Geometry check sheet. Reference: the model listing, model coordinates, mm. A direction names the side the tool comes from. Round coordinates to 2 decimals unless told otherwise and drop trailing zeros. Order: outer loops, then holes, each group sorted by start corner. A loop starts at its lowest first (then second) coordinate and runs counter-clockwise, first axis right, second up.
```python
from build123d import *

# Parameters (mm, degrees)
F0_W      = 1663.7
F0_H      = 304.8
F1_DEPTH  = 19.05
F2_W      = 50.8
F2_H      = 19.05
F3_DEPTH  = 304.8
F4_W      = 1308.1
F4_H      = 19.05
F5_DEPTH  = 304.8
F7_DEPTH  = 19.05
F8_DEPTH  = 19.05
F9_DEPTH  = 19.05
F11_DEPTH = 19.05
F12_W     = 276.225
F12_H     = 19.05
F13_DEPTH = 304.8
F14_DEPTH = 50.8
F15_DEPTH = 304.8
F16_DEPTH = 304.8
F17_W     = 304.8
F17_H     = 19.05
F18_DEPTH = 152.4


with BuildPart() as f1:
    # F0 (on Front) → F1 (new body)
    with BuildSketch(Plane.XZ):
        Rectangle(F0_W, F0_H)
    extrude(amount=F1_DEPTH)

    # F2 (on face) → F3 (join)
    with BuildSketch(Plane.XZ.offset(19.05)):
        with Locations((806.45, -142.113)):
            Rectangle(F2_W, F2_H)
    extrude(amount=F3_DEPTH)

    # F4 (on face) → F5 (join)
    with BuildSketch(Plane.XZ.offset(19.05)):
        with Locations((-177.8, -142.113)):
            Rectangle(F4_W, F4_H)
    extrude(amount=F5_DEPTH)

    # F6 (on face) → F7 (join)
    with BuildSketch(Plane.XZ.offset(323.85)):
        Polygon((-831.85, 152.4), (-831.85, -151.638), (-831.85, -152.4), (831.85, -152.4), (831.85, 152.4), align=None)
    extrude(amount=F7_DEPTH)

    # F8 (cut): a face of the model
    f8_faces = [f1.faces().sort_by_distance(p)[0] for p in [
        (0, -333.375, 152.4),
    ]]
    extrude(f8_faces, amount=-F8_DEPTH, mode=Mode.SUBTRACT)

    # F9 (cut): a face of the model
    f9_faces = [f1.faces().sort_by_distance(p)[0] for p in [
        (0, -9.525, 152.4),
    ]]
    extrude(f9_faces, amount=-F9_DEPTH, mode=Mode.SUBTRACT)

    # F10 (on face) → F11 (join)
    with BuildSketch(Plane.XY.offset(133.35)):
        Polygon((831.85, -393.7), (831.85, -342.9), (831.85, -323.85), (831.85, -19.05), (781.05, -19.05), (781.05, -323.85), (425.45, -323.85), (425.45, -19.05), (361.95, -19.05), (361.95, -323.85), (-615.95, -323.85), (-679.45, -323.85), (-831.85, -323.85), (-831.85, -393.7), align=None)
        Polygon((781.05, -19.05), (831.85, -19.05), (831.85, 50.8), (-831.85, 50.8), (-831.85, -19.05), (-679.45, -19.05), (-679.45, -323.85), (-615.95, -323.85), (-615.95, -19.05), (361.95, -19.05), (425.45, -19.05), align=None)
    extrude(amount=F11_DEPTH)

    # F12 (on face) → F13 (join)
    with BuildSketch(Plane(origin=(0, -323.85, 0), x_dir=(-1, 0, 0), z_dir=(0, 1, 0))):
        with Locations((-617.5375, -142.113)):
            Rectangle(F12_W, F12_H)
    extrude(amount=F13_DEPTH)

    # F14 (cut): a face of the model
    f14_faces = [f1.faces().sort_by_distance(p)[0] for p in [
        (-831.85, -329.2396501742, 9.906),
    ]]
    extrude(f14_faces, amount=-F14_DEPTH, mode=Mode.SUBTRACT)

    # F15 (add): a face of the model
    f15_faces = [f1.faces().sort_by_distance(p)[0] for p in [
        (831.85, -329.2396501742, -152.019),
    ]]
    extrude(f15_faces, amount=F15_DEPTH)

    # F16 (cut): a face of the model
    f16_faces = [f1.faces().sort_by_distance(p)[0] for p in [
        (781.05, -171.45, 142.875),
    ]]
    extrude(f16_faces, amount=-F16_DEPTH, mode=Mode.SUBTRACT)

    # F17 (on face) → F18 (cut)
    with BuildSketch(Plane(origin=(-781.05, 0, 0), x_dir=(0, -1, 0), z_dir=(-1, 0, 0))):
        with Locations((171.45, -142.113)):
            Rectangle(F17_W, F17_H)
    extrude(amount=-F18_DEPTH, mode=Mode.SUBTRACT)


solid = f1.part
```
(1) Draft check along Y on faces 1 (the flat face through (956, -169, -132.588)), 2 (the flat face through (164, 0, -12)). Enter one of: released by +Y, released by -Y, zero draft, split by the parting line, or undercut.
Returned:
face 1: undercut
face 2: released by +Y
(2) Set-up check for faces 3 (the flat face through (-648, -169, 133.35)), 4 (the flat face through (-781.05, -2, 22)), 5 (the flat face through (164, -342.9, -12)), 6 (the flat face through (164, 25, 133.35)), 7 (the flat face through (619, -174, -132.588)): record each of +Z, -Z, +X, -X, +Y, -Y from which the full face is reachable in a straight line by a thin tool's end or side.
Returned:
face 3: +X, -X
face 4: +Z, -Z, -X, +Y, -Y
face 5: -Z, +X, -X, -Y
face 6: -Z, +X, -X, +Y
face 7: +Z, +X, -X
(3) Material ranges on line 1 (Y direction, x = -546, z = -29.5); line 2 (Z direction, x = 899, y = -307); line 3 (Z direction, x = -666, y = 23.5), recorded low to high.
Returned:
line 1: y = -342.9 to -323.85, -19.05 to 0
line 2: z = -151.64 to -132.59
line 3: z = 133.35 to 152.4
(4) Depth check by flat-ended pin: P1, Ø19, axis at x = 388.5, y = -160.5, coming from the -Z side; P2, Ø15, axis at y = -166.5, z = -144.5, coming from the -X side; P3, Ø8, axis at x = 130.5, z = -3, coming from the -Y side. Enter the tip coordinate at first touch or a pass-through.
Returned:
P1: stops at z = -151.64
P2: stops at x = -628.65
P3: stops at y = -342.9
(5) Sectioned sample at C-C, the plane x = 384. Record the cut outline in (y, z).
Returned:
outline: (-393.7, 133.35) - (-342.9, 133.35) - (-342.9, -152.4) - (-323.85, -152.4) - (-323.85, -151.64) - (-19.05, -151.64) - (-19.05, -152.4) - (0, -152.4) - (0, 133.35) - (50.8, 133.35) - (50.8, 152.4) - (-393.7, 152.4) - close; hole (-323.85, -132.59) - (-19.05, -132.59) - (-19.05, 133.35) - (-323.85, 133.35) - close
(6) Sectioned sample at A-A, the plane y = -134. Record the cut outline in (x, z) (3 decimals), and give its area (3 significant figures).
Returned:
outline: (-679.45, 133.35) - (-615.95, 133.35) - (-615.95, 152.4) - (-679.45, 152.4) - close; (-628.65, -151.638) - (476.25, -151.638) - (476.25, -132.588) - (-628.65, -132.588) - close; (361.95, 133.35) - (425.45, 133.35) - (425.45, 152.4) - (361.95, 152.4) - close; (479.425, -151.638) - (755.65, -151.638) - (755.65, -132.588) - (479.425, -132.588) - close; (781.05, -151.638) - (1136.65, -151.638) - (1136.65, -132.588) - (781.05, -132.588) - close; (1085.85, 133.35) - (1136.65, 133.35) - (1136.65, 152.4) - (1085.85, 152.4) - close
area: 36,500 mm2
(7) Sectioned sample at B-B, the plane z = -20.5. Record the cut outline in (x, y), and give its area (3 significant figures).
Returned:
outline: (-781.05, -342.9) - (1136.65, -342.9) - (1136.65, -323.85) - (-781.05, -323.85) - close; (-781.05, -19.05) - (1136.65, -19.05) - (1136.65, 0) - (-781.05, 0) - close
area: 73,100 mm2
